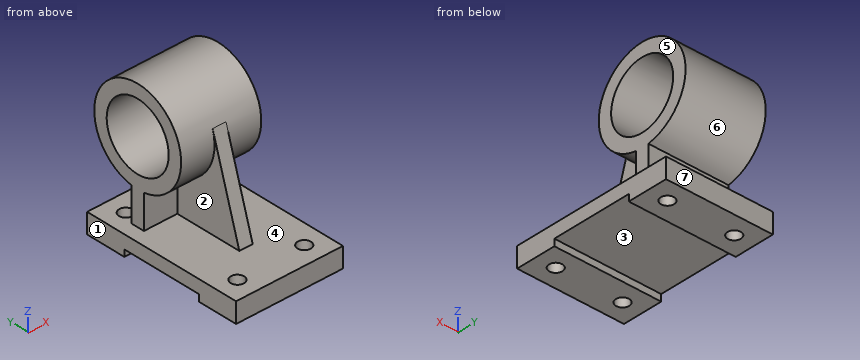
Solid Edge part; units mm, degrees
sketch "Sketch1" plane through (0, 0, 0) normal (1, 0, 0) x (0, 1, 0)
  line L0 (60, 10) -> (-60, 10)
  line L1 (-60, 10) -> (-60, -5)
  line L2 (-60, -5) -> (-30, -5)
  line L3 (-30, -5) -> (-30, 0)
  line L4 (-30, 0) -> (0, 0)
  line L5 (0, 0) -> (30, 0)
  line L6 (30, 0) -> (30, -5)
  line L7 (30, -5) -> (60, -5)
  line L8 (60, -5) -> (60, 10)
extrude "Protrusion1" add sketch "Sketch1" along normal mid plane 80
sketch "Sketch2" plane through (0, 0, 10) normal (0, 0, 1) x (1, 0, 0)
  circle A0 centre (-25, -45) radius 5
  circle A1 centre (25, -45) radius 5
  circle A2 centre (25, 45) radius 5
  circle A3 centre (-25, 45) radius 5
extrude "ExtrudedCutout_1" cut sketch "Sketch2" against normal blind 41.1924
sketch "Sketch3" plane through (0, 0, 0) normal (1, 0, 0) x (0, 1, 0)
  line L0 (35, 35.359) -> (35, 10)
  line L1 (35, 10) -> (25, 10)
  line L2 (25, 10) -> (25, 35.359)
  arc A0 (25, 35.359) -> (35, 35.359) centre (30, 70) cw
  circle A1 centre (30, 70) radius 25
extrude "ExtrudedProtrusion_2" add sketch "Sketch3" along normal mid plane 60
sketch "Sketch4" plane through (0, 0, 0) normal (1, 0, 0) x (0, 1, 0)
  line L0 (-25, 10) -> (-3.4631, 80.2578)
  line L1 (24.641, 10) -> (24.641, 35.4127)
  line L2 (-25, 10) -> (24.641, 10)
  arc A0 (24.641, 35.4127) -> (-3.4631, 80.2578) centre (30, 70) cw
extrude "ExtrudedProtrusion_3" add sketch "Sketch4" along normal mid plane 10
Design review of the part built by this model. Coordinates are the model's own, in mm. Face numbers are marked on the shaded views. A direction names the side the tool comes from. Round coordinates to 2 decimals unless told otherwise and drop trailing zeros. Write each loop counter-clockwise with the first axis right and the second up, starting at its lowest first coordinate (ties: lowest second). Pieces come first, ordered by that corner, then holes.
Item 1: We need section D-D on y = 21. Write out the cut boundary in (x, z).
Item 2: For probe 1 along Y at (x, z) = (25, 1.5); probe 2 along Y at (x, z) = (6.5, 70.5) (3 decimals); probe 3 along X at (y, z) = (20, 20), list the stretches that pass through material, from the lowest coordinate up.
Item 3: For the marked faces 5, 6 and 7, list the 3-axis set-ups (+Z, -Z, +X, -X, +Y, -Y) from which the entire face can be reached by the end or side of a thin tool; tool diameter is ignored.
Item 4: We need section A-A on x = -22. Write out the cut boundary in (y, z), and give its area (3 significant figures).
Item 5: Clearance check with flat-ended pins moving along their axes: pin 1 Ø12.5 at (x, z) = (-14.5, 20) entering from +Y; pin 2 Ø5.5 at (x, z) = (-6.5, -2.5) entering from +Y; pin 3 Ø6 at (x, y) = (20, 45.5) entering from +Z. State where each tip first meets the part, or that it passes through.
Item 6: We need section B-B on y = -45. Write out the cut boundary in (x, z).
Item 7: The part is to be moulded in two halves that separate along Z. For the marked faces 1, 2, 3 and 4, say which applies: +Z half, -Z half, draft (parallel to the pull), parting line (faces both ways), or undercut.
Item 8: We need section C-C on z = 52. Write out the cut boundary in (x, y), and give its area (3 significant figures).
Returned:
1. outline: (-40, 0) - (40, 0) - (40, 10) - (5, 10) - (5, 36.18) - (30, 36.18) - (30, 46.68) - (-30, 46.68) - (-30, 36.18) - (-5, 36.18) - (-5, 10) - (-40, 10) - close; (-30, 93.32) - (30, 93.32) - (30, 103.82) - (-30, 103.82) - close
2. probe 1: y = -60 to -50, -40 to 40, 50 to 60
2. probe 2: y = -4.996 to 5.005, 54.995 to 64.996
2. probe 3: x = -5 to 5
3. face 5: +Z, +X, +Y, -Y
3. face 6: none
3. face 7: -Z, +X, -X, +Y
4. outline: (-60, -5) - (-49, -5) - (-49, 10) - (-60, 10) - close; (-41, -5) - (-30, -5) - (-30, 0) - (30, 0) - (30, -5) - (41, -5) - (41, 10) - (35, 10) - (35, 35.36) arc R35 ccw (long way) to (25, 35.36) - (25, 10) - (-41, 10) - close; (49, -5) - (60, -5) - (60, 10) - (49, 10) - close; hole circle Ø50 at (30, 70)
4. area: 3,400 mm2
5. pin 1: stops at y = 35
5. pin 2: stops at y = 60
5. pin 3: stops at z = 102.69
6. outline: (-40, -5) - (-30, -5) - (-30, 10) - (-40, 10) - close; (-20, -5) - (20, -5) - (20, 10) - (-20, 10) - close; (30, -5) - (40, -5) - (40, 10) - (30, 10) - close
7. face 1: draft
7. face 2: undercut
7. face 3: -Z half
7. face 4: undercut
8. outline: (-30, -0.02) - (-5, -0.02) - (-5, -12.13) - (5, -12.13) - (5, -0.02) - (30, -0.02) - (30, 12.65) - (-30, 12.65) - close; (-30, 47.35) - (30, 47.35) - (30, 60.02) - (-30, 60.02) - close
8. area: 1,640 mm2
